For this review, use the dimensioned drawing (mm, ordinates from the lowest corner) and the shaded views. A direction names the side the tool comes from. Round coordinates to 2 decimals unless told otherwise and drop trailing zeros. Order: outer loops, then holes, each group sorted by start corner. A loop starts at its lowest first (then second) coordinate and runs counter-clockwise, first axis right, second up. Notation, with made-up numbers: M 33.25,6 L 81.25,6 A10 cw 81.25,10 Z; hole C 77,69.5 d3. An arc over 180 degrees is marked long. Use a Markdown table: item, result. Add a question column.
1. Consider section A-A on z = 35. State the section outline as (x, y) points.
2. To check wall thickness, follow probe 1 along X at (y, z) = (16, 35); probe 2 along X at (y, z) = (29, 58.5); probe 3 along X at (y, z) = (21.5, 125.5). State the ranges of each line that lie inside material, in increasing order.
3. For the marked faces 1, 2 and 3, list the 3-axis set-ups (+Z, -Z, +X, -X, +Y, -Y) from which the entire face can be reached by the end or side of a thin tool; tool diameter is ignored.
4. Consider section C-C on x = 56. State the section outline as (y, z) points, then the cut area to 3 significant figures.
5. Consider section B-B on y = 22. State the section outline as (x, z) points (1 decimal).
6. Insertion check: P1, Ø3, axis at y = 9.5, z = 99, coming from the -X side; P2, Ø12, axis at x = 84, y = 20.5, coming from the -Z side; P3, Ø4, axis at x = 22, y = 18.5, coming from the -Z side. Each pin has a flat end and moves straight along its axis. Give the tip position at first contact, or say it passes through.
7. Consider section D-D on z = 12. State the section outline as (x, y) points.
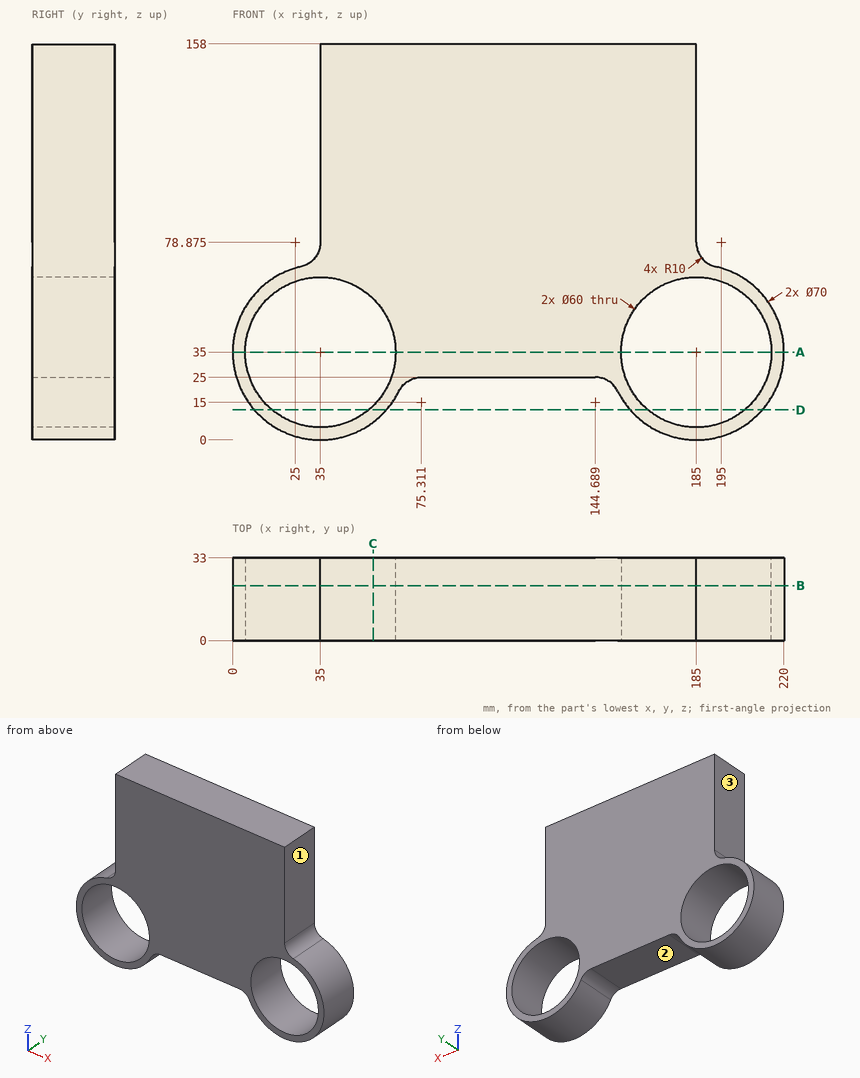
Answer block:
| question | item | result |
|---|---|---|
| 1 | outline | M 0,0 L 5,0 L 5,33 L 0,33 Z; M 65,0 L 155,0 L 155,33 L 65,33 Z; M 215,0 L 220,0 L 220,33 L 215,33 Z |
| 2 | probe 1 | 0 to 5, 65 to 155, 215 to 220 |
| 2 | probe 2 | 9.06 to 16.35, 53.65 to 166.35, 203.65 to 210.94 |
| 2 | probe 3 | 35 to 185 |
| 3 | face 1 | +Z, +X, +Y, -Y |
| 3 | face 2 | -Z, +Y, -Y |
| 3 | face 3 | +Z, -X, +Y, -Y |
| 4 | outline | M 0,7 L 33,7 L 33,13.58 L 0,13.58 Z; M 0,56.42 L 33,56.42 L 33,158 L 0,158 Z |
| 4 | area | 3,570 mm^2 |
| 5 | outline | M 27.2,69.1 A35 ccw long 66.4,19.4 A10 cw 75.3,25 L 144.7,25 A10 cw 153.6,19.4 A35 ccw long 192.8,69.1 A10 cw 185,78.9 L 185,158 L 35,158 L 35,78.9 A10 cw Z; hole C 35,35 d60; hole C 185,35 d60 |
| 6 | P1 | x = 35 |
| 6 | P2 | z = 25 |
| 6 | P3 | z = 1.77 |
| 7 | outline | M 8.62,0 L 15.74,0 L 15.74,33 L 8.62,33 Z; M 54.26,0 L 61.38,0 L 61.38,33 L 54.26,33 Z; M 158.62,0 L 165.74,0 L 165.74,33 L 158.62,33 Z; M 204.26,0 L 211.38,0 L 211.38,33 L 204.26,33 Z |
